Here's how the part is built. I have some questions about the finished solid (model axes, mm). Give positions to 0.01 mm unless a question says otherwise; leave off trailing zeros. Order: outer loops, then holes, each group sorted by start corner. A loop starts at its lowest first (then second) coordinate and runs counter-clockwise, first axis right, second up. Notation, with made-up numbers: M -33.75,62.5 L 12.25,62.5 A17 ccw 12.25,78.5 Z; hole C 10,-27.75 d10. An arc over 180 degrees is marked long. Use one line per item in the form item = value.
from build123d import *

# Parameters (mm, degrees)
F0_R     = 1.651
F1_DEPTH = 3.175


with BuildPart() as f1:
    # F0 (on Front) → F1 (new body)
    with BuildSketch(Plane.XZ):
        with BuildLine():
            Line((-91.7235008659, -10.6519622226), (-182.5513082058, -73.0949387128))
            ThreePointArc((-182.5513082058, -73.0949387128), (-187.3498879631, -96.5075485814), (-170.466153763, -113.4225179282))
            ThreePointArc((-170.466153763, -113.4225179282), (-36.1095650791, -104.4974979583), (98.0233131029, -116.3178149951))
            Line((98.0233131029, -116.3178149951), (108.933846237, -116.3178149951))
            ThreePointArc((108.933846237, -116.3178149951), (110.7304402005, -106.6101038659), (108.933846237, -96.9023927367))
            Line((108.933846237, -96.9023927367), (108.933846237, -83.3431183613))
            Line((108.933846237, -83.3431183613), (80.270888986, 46.2421850049))
            Line((80.270888986, 46.2421850049), (35.8280335171, 41.0442404951))
            Line((35.8280335171, 41.0442404951), (-91.7235008659, -10.6519622226))
        make_face()
        with Locations((-168.5793250799, -105.0686376895)):
            Circle(F0_R, mode=Mode.SUBTRACT)
        with Locations((-145.6571504202, -92.9395344899)):
            Circle(F0_R, mode=Mode.SUBTRACT)
        with Locations((-123.6779055701, -81.3093757901)):
            Circle(F0_R, mode=Mode.SUBTRACT)
        with Locations((-92.9428839156, -65.04616102)):
            Circle(F0_R, mode=Mode.SUBTRACT)
        with Locations((-57.7850724394, -46.4426589528)):
            Circle(F0_R, mode=Mode.SUBTRACT)
        with Locations((106.6226363182, -112.6031056046)):
            Circle(F0_R, mode=Mode.SUBTRACT)
        Polygon((29.4560794945, -59.7358805891), (32.0242086794, -60.2470721804), (31.8355546398, -61.2572841346), (24.8736120152, -61.2572841346), (25.0622660549, -60.2470721804), (27.1922310187, -59.7358805891), (40.1667604553, -35.5455642146), (43.7937865079, -35.5455642146), (48.5527367984, -59.7358805891), (50.9261263295, -60.2470721804), (50.7192154473, -61.2572841346), (41.6881640008, -61.2572841346), (41.895074883, -60.2470721804), (44.6153444225, -59.7358805891), (43.3982215861, -52.3783730427), (33.3569581853, -52.3783730427), align=None, mode=Mode.SUBTRACT)
        Polygon((60.760478848, -34.2310715512), (56.251038739, -59.9245346287), (59.2390753025, -60.3992125349), (59.0869349479, -61.2572841346), (52.8674372537, -61.2572841346), (57.3707917485, -35.5455642146), (54.9182892331, -35.0891431509), (55.0704295876, -34.2310715512), align=None, mode=Mode.SUBTRACT)
        Polygon((71.5807008641, -34.2310715512), (67.0712607551, -59.9245346287), (70.0592973185, -60.3992125349), (69.907156964, -61.2572841346), (63.6876592697, -61.2572841346), (68.1910137646, -35.5455642146), (65.7385112491, -35.0891431509), (65.8906516037, -34.2310715512), align=None, mode=Mode.SUBTRACT)
        Polygon((80.8977761772, -43.3777496671), (77.988852598, -59.9245346287), (80.9708035473, -60.3992125349), (80.8186631928, -61.2572841346), (74.5991654985, -61.2572841346), (77.5080890776, -44.7104991731), (75.0555865622, -44.2358212668), (75.2077269167, -43.3777496671), align=None, mode=Mode.SUBTRACT)
        with BuildLine():
            add(Edge.make_bspline(
                [(81.4637382961, -36.0750126484), (82.0722997143, -36.6835740667), (82.0722997143, -37.5416456664)],
                knots=[0, 0, 0, 1, 1, 1], degree=2))
            add(Edge.make_bspline(
                [(82.0722997143, -37.5416456664), (82.0722997143, -38.3814604235), (81.4637382961, -38.9900218417)],
                knots=[0, 0, 0, 1, 1, 1], degree=2))
            add(Edge.make_bspline(
                [(81.4637382961, -38.9900218417), (80.8551768779, -39.59858326), (80.0031908924, -39.59858326)],
                knots=[0, 0, 0, 1, 1, 1], degree=2))
            add(Edge.make_bspline(
                [(80.0031908924, -39.59858326), (79.1633761352, -39.59858326), (78.554814717, -38.9900218417)],
                knots=[0, 0, 0, 1, 1, 1], degree=2))
            add(Edge.make_bspline(
                [(78.554814717, -38.9900218417), (77.9462532988, -38.3814604235), (77.9462532988, -37.5416456664)],
                knots=[0, 0, 0, 1, 1, 1], degree=2))
            add(Edge.make_bspline(
                [(77.9462532988, -37.5416456664), (77.9462532988, -36.6835740667), (78.554814717, -36.0750126484)],
                knots=[0, 0, 0, 1, 1, 1], degree=2))
            add(Edge.make_bspline(
                [(78.554814717, -36.0750126484), (79.1633761352, -35.4664512302), (80.0031908924, -35.4664512302)],
                knots=[0, 0, 0, 1, 1, 1], degree=2))
            add(Edge.make_bspline(
                [(80.0031908924, -35.4664512302), (80.8551768779, -35.4664512302), (81.4637382961, -36.0750126484)],
                knots=[0, 0, 0, 1, 1, 1], degree=2))
        make_face(mode=Mode.SUBTRACT)
        with Locations((-22.6272609633, -27.8391568856)):
            Circle(F0_R, mode=Mode.SUBTRACT)
        with Locations((8.1077606912, -11.5759421154)):
            Circle(F0_R, mode=Mode.SUBTRACT)
        with Locations((25.8241575211, 5.8733294718)):
            Circle(F0_R, mode=Mode.SUBTRACT)
        with Locations((32.8517727122, 20.2778487448)):
            Circle(F0_R, mode=Mode.SUBTRACT)
    extrude(amount=F1_DEPTH)


solid = f1.part
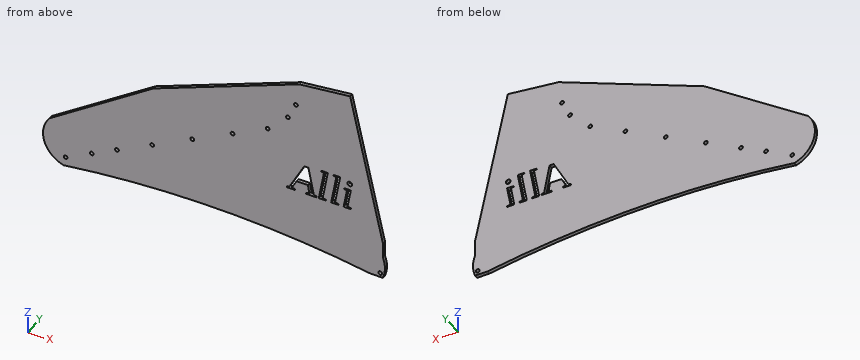
Q1. I want a section at C-C on y = -1.3. State how many separate pieces and enclosed holes the cut face has, then the cut area to 3 significant figures.
Found:
separate_pieces = 1
enclosed_holes = 15
area = 30,700 mm²
Q2. I want a section at B-B on z = 31. Write out the boundary of the cut face in (x, y) (3 decimals), then the cut area to 3 significant figures.
Found:
outline = M 11.046,-3.175 L 83.642,-3.175 L 83.642,0 L 11.046,0 Z
area = 230 mm²
Q3. I need wall thicknesses on L1, parallel to X at y = -2.6, z = -55; L2, parallel to X at y = -1.6, z = -51; L3, parallel to X at y = -0.5, z = -93. Which ranges of each line are inside material? Lowest first, please.
Found:
L1 = -156.23 to 29.73, 31.97 to 43.83, 47.62 to 53.96, 57.12 to 64.78, 67.94 to 75.7, 78.85 to 102.66
L2 = -150.41 to 31.88, 46.83 to 54.66, 57.82 to 65.48, 68.64 to 76.4, 79.56 to 101.78
L3 = -188.13 to -147.31, -144.01 to 108.93
Q4. I want a section at A-A on x = -103. Write out the boundary of the cut face in (y, z) (3 decimals).
Found:
outline = M -3.175,-106.338 L 0,-106.338 L 0,-18.404 L -3.175,-18.404 Z
Q5. I'm going to push flat-ended pins straight in: pin 1 Ø1 at (x, y) = (44.5, -1) entering from +Z; pin 2 Ø1 at (x, y) = (68, -1) entering from -Z; pin 3 Ø10 at (x, z) = (46, -85) entering from +Y; pin 4 Ø1.6 at (x, y) = (57, -1.5) entering from -Z. Where does each tip first touch, or does it pass through?
Found:
pin_1 = 42.12
pin_2 = -111.92
pin_3 = 0
pin_4 = -110.58
